from build123d import *

# Parameters (mm, degrees)
SKETCH1_W               = 39.6
SKETCH1_H               = 59.6
BOSS_EXTRUDE1_DEPTH     = 25
CUT_EXTRUDE1_DEPTH      = 5
CUT_EXTRUDE2_DEPTH      = 44.647222134
CUT_EXTRUDE2_DEPTH_BACK = 44.647222134
SKETCH3_R               = 2.75
CUT_EXTRUDE4_START      = 25
CUT_EXTRUDE4_DEPTH      = 5


with BuildPart() as part:
    # Sketch1 → Boss-Extrude1 (new body)
    with BuildSketch(Plane(origin=(0, 0, 0), x_dir=(0, 0, -1), z_dir=(1, 0, 0))):
        Rectangle(SKETCH1_W, SKETCH1_H)
    extrude(amount=BOSS_EXTRUDE1_DEPTH)

    # Sketch2 → Cut-Extrude1 (cut)
    with BuildSketch(Plane(origin=(0, 0, 0), x_dir=(0, 0, -1), z_dir=(1, 0, 0))):
        Polygon((4.67653718, 10), (2.33826859, 14.05), (-2.33826859, 14.05), (-4.67653718, 10), (-2.33826859, 5.95), (2.33826859, 5.95), align=None)
    extrude(amount=CUT_EXTRUDE1_DEPTH, mode=Mode.SUBTRACT)

    # Sketch3 → Cut-Extrude2 (cut, two sides: drawn at the far end of the back side and taken through both)
    with BuildSketch(Plane(origin=(0, 0, 0), x_dir=(0, 0, -1), z_dir=(1, 0, 0)).offset(-CUT_EXTRUDE2_DEPTH_BACK)):
        with Locations((0, 10)):
            Circle(SKETCH3_R)
    extrude(amount=CUT_EXTRUDE2_DEPTH + CUT_EXTRUDE2_DEPTH_BACK, mode=Mode.SUBTRACT)

    # Sketch2<2> → Cut-Extrude4 (cut)
    with BuildSketch(Plane(origin=(0, 0, 0), x_dir=(0, 0, -1), z_dir=(1, 0, 0)).offset(CUT_EXTRUDE4_START)):
        Polygon((4.67653718, 10), (2.33826859, 14.05), (-2.33826859, 14.05), (-4.67653718, 10), (-2.33826859, 5.95), (2.33826859, 5.95), align=None)
    extrude(amount=-CUT_EXTRUDE4_DEPTH, mode=Mode.SUBTRACT)


solid = part.part
Build history of the part. All positions in model axes, mm. A direction names the side the tool comes from. Give positions to 0.01 mm unless a question says otherwise; leave off trailing zeros. Order: outer loops, then holes, each group sorted by start corner. A loop starts at its lowest first (then second) coordinate and runs counter-clockwise, first axis right, second up. Notation, with made-up numbers: M 51.25,35.25 L 83.25,35.25 A16 cw 83.25,42.25 Z; hole C 5,32.5 d5. An arc over 180 degrees is marked long. Use one line per item in the form item = value.
1) Saw through at C-C (y = 8.5). Give the cut face in (x, z), plus the area to 3 significant figures.
Calculated:
outline = M 0,-19.8 L 25,-19.8 L 25,-3.81 L 20,-3.81 L 20,-2.3 L 5,-2.3 L 5,-3.81 L 0,-3.81 Z; M 0,3.81 L 5,3.81 L 5,2.3 L 20,2.3 L 20,3.81 L 25,3.81 L 25,19.8 L 0,19.8 Z
area = 845 mm2
2) Probe probe 1 along Z at (x, y) = (10, 10); probe 2 along Y at (x, z) = (12.5, 0); probe 3 along Z at (x, y) = (9, 8). List the from-to ranges inside material, lowest first.
Calculated:
probe_1 = -19.8 to -2.75, 2.75 to 19.8
probe_2 = -29.8 to 7.25, 12.75 to 29.8
probe_3 = -19.8 to -1.89, 1.89 to 19.8
3) Tool access for faces 1 (the face through (2, 5.95, 0)), 2 (the face through (23, 5.95, 0)), 3 (the face through (0, 0, 0)): list every direction of +Z, -Z, +X, -X, +Y, -Y with a clear straight run to the whole face (end or side of a thin tool).
Calculated:
face_1 = -X
face_2 = +X
face_3 = +Z, -Z, -X, +Y, -Y
4) Saw through at A-A (x = 22.5). Give the cut face in (y, z).
Calculated:
outline = M -29.8,-19.8 L 29.8,-19.8 L 29.8,19.8 L -29.8,19.8 Z; hole M 5.95,-2.34 L 10,-4.68 L 14.05,-2.34 L 14.05,2.34 L 10,4.68 L 5.95,2.34 Z
5) Saw through at B-B (z = 0). Give the cut face in (x, y), plus the area to 3 significant figures.
Calculated:
outline = M 0,-29.8 L 25,-29.8 L 25,5.95 L 20,5.95 L 20,7.25 L 5,7.25 L 5,5.95 L 0,5.95 Z; M 0,14.05 L 5,14.05 L 5,12.75 L 20,12.75 L 20,14.05 L 25,14.05 L 25,29.8 L 0,29.8 Z
area = 1,330 mm2
6) Two-plate mould, pull along Z, no slides. Class faces 4 (the face through (20, 13, 0)), 5 (the face through (12, 29.8, 0)): released by +Z, released by -Z, zero draft, split by the parting line, or undercut.
Calculated:
face_4 = undercut
face_5 = zero draft
